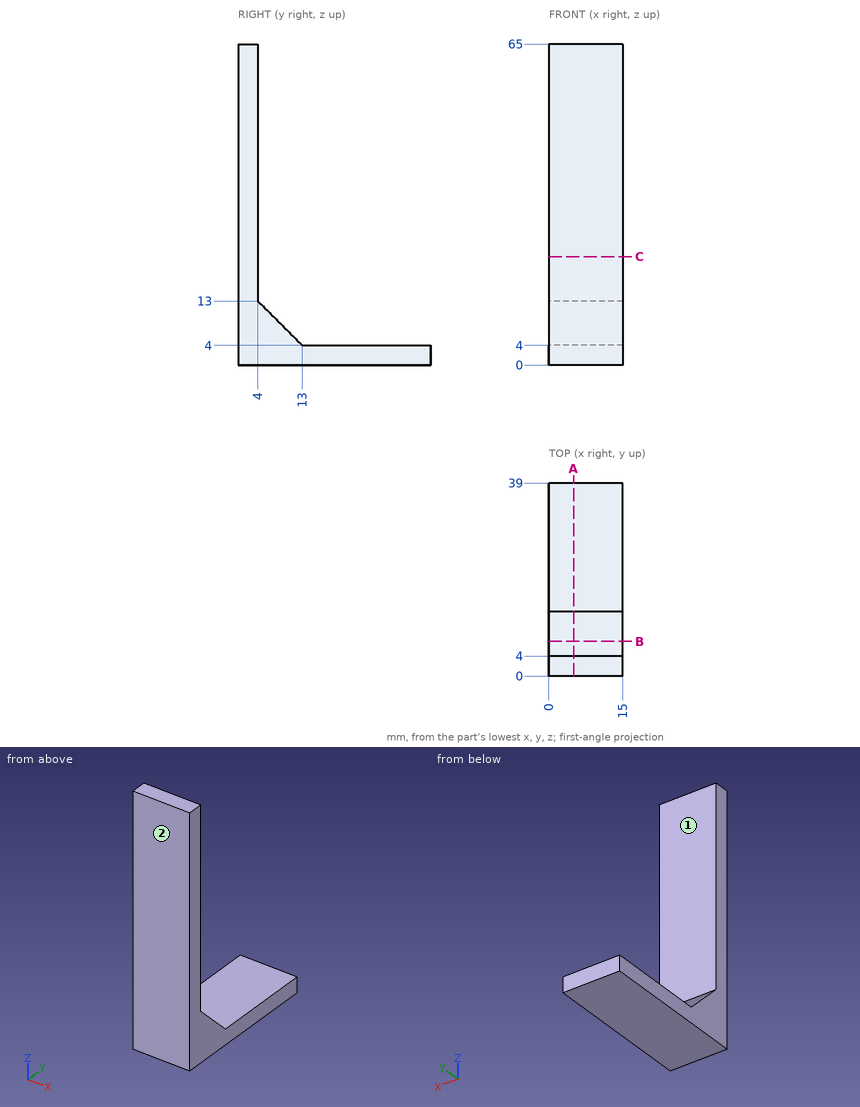
For this review, use the dimensioned drawing (mm, ordinates from the lowest corner) and the shaded views. A direction names the side the tool comes from. Coordinates: 2 decimals unless noted, no trailing zeros. Loops run counter-clockwise (first coordinate to the right, second up) from the corner with the lowest first, then second, coordinate; pieces in that order, holes last.
1. For the marked faces 1 and 2, list the 3-axis set-ups (+Z, -Z, +X, -X, +Y, -Y) from which the entire face can be reached by the end or side of a thin tool; tool diameter is ignored.
2. Insertion check: P1, Ø1.5, axis at x = 8.5, z = 56, coming from the -Y side; P2, Ø5, axis at x = 9, y = 13.5, coming from the +Z side; P3, Ø1, axis at x = 5, y = 6, coming from the +Z side; P4, Ø4.5, axis at x = 9.5, y = 28, coming from the +Z side. Each pin has a flat end and moves straight along its axis. Give the tip position at first contact, or say it passes through.
3. Add section C-C, the plane z = 22. Give the boundary of the cut face in (x, y).
4. Add section B-B, the plane y = 7. Give the boundary of the cut face in (x, z), then the cut area to 3 significant figures.
5. For line 1 (Z direction, x = 4.5, y = 33.5); line 2 (Y direction, x = 6.5, z = 10.5), list the stretches that pass through material, from the lowest coordinate up.
6. Add section A-A, the plane x = 5. Give the boundary of the cut face in (y, z), then the cut area to 4 significant figures.
Result:
1. face 1: +Z, +X, -X, +Y
1. face 2: +Z, -Z, +X, -X, -Y
2. P1: stops at y = 0
2. P2: stops at z = 6
2. P3: stops at z = 11.5
2. P4: stops at z = 4
3. outline: (0, 0) - (15, 0) - (15, 4) - (0, 4) - close
4. outline: (0, 0) - (15, 0) - (15, 10) - (0, 10) - close
4. area: 150 mm2
5. line 1: z = 0 to 4
5. line 2: y = 0 to 6.5
6. outline: (0, 0) - (39, 0) - (39, 4) - (13, 4) - (4, 13) - (4, 65) - (0, 65) - close
6. area: 440.5 mm2
